from build123d import *

# Parameters (mm, degrees)
BOSS_EXTRUDE2_DEPTH = 10
SKETCH2_R           = 4
CUT_EXTRUDE1_DEPTH  = 10


with BuildPart() as part:
    # Sketch1 → Boss-Extrude2 (new body)
    with BuildSketch(Plane.XY):
        Polygon((0, 25.51264103), (0, 30), (1.000891574, 30), (10.376925968, 23.306957325), (12.202099292, 27.406363729), (13.116459243, 26.99926445), (18.959587166, 17.071288962), (22.294344764, 20.073918191), (22.96407195, 19.330110797), (24.263963499, 7.88383965), (28.531695489, 9.270509831), (28.840987995, 8.318605378), (25.372880113, -2.666797161), (29.835656861, -3.135853898), (29.731035203, -4.131262483), (22.094595249, -12.756320515), (25.980762114, -15), (25.480316326, -15.86679753), (14.995954144, -20.640160164), (17.633557569, -24.270509831), (16.823819276, -24.858819138), (5.304376334, -24.955128612), (6.237350725, -29.344428022), (5.258331033, -29.552525082), (-5.304376334, -24.955128612), (-6.237350725, -29.344428022), (-7.216370416, -29.136330963), (-14.995954144, -20.640160164), (-17.633557569, -24.270509831), (-18.443295862, -23.682200525), (-22.094595249, -12.756320515), (-25.980762114, -15), (-26.481207901, -14.13320247), (-25.372880113, -2.666797161), (-29.835656861, -3.135853898), (-29.940278519, -2.140445313), (-24.263963499, 7.88383965), (-28.531695489, 9.270509831), (-28.222402983, 10.222414285), (-18.959587165, 17.071288962), (-22.294344764, 20.073918191), (-21.624617578, 20.817725585), (-10.376925968, 23.306957325), (-12.202099292, 27.406363729), (-11.287739341, 27.813463008), align=None)
    extrude(amount=BOSS_EXTRUDE2_DEPTH)

    # Sketch2 → Cut-Extrude1 (cut)
    with BuildSketch(Plane(origin=(0, 0, 0), x_dir=(-1, 0, 0), z_dir=(0, 0, -1))):
        Circle(SKETCH2_R)
    extrude(amount=-CUT_EXTRUDE1_DEPTH, mode=Mode.SUBTRACT)


solid = part.part
The listing builds one solid part. Answer for the finished solid, in the listing's coordinates (mm). A direction names the side the tool comes from. Give positions to 0.01 mm unless a question says otherwise; leave off trailing zeros. Order: outer loops, then holes, each group sorted by start corner. A loop starts at its lowest first (then second) coordinate and runs counter-clockwise, first axis right, second up. Notation, with made-up numbers: (-35, 54) - (-16, 54) arc R24 cw to (-16, 72) - close; hole circle Ø8 at (68.25, 87). An arc over 180 degrees is marked (long way). Answer as CSV lines item,"result".
Q1. Determine the mould class of faces 1 (the face through (11.277, 25.328, 4.93)), 2 (the face through (0.051, -27.286, 4.93)), 3 (the face through (-11.277, 25.328, 4.93)), 4 (the face through (0, 28, 5)) for opening direction Y: pulls with the +Y half, pulls with the -Y half, needs draft (parallel to the pull), parting line crosses it, or undercut.
Answer key:
face 1,"pulls with the +Y half"
face 2,"pulls with the -Y half"
face 3,"undercut"
face 4,"needs draft"
Q2. A cutting plane is placed at A-A, the plane x = 16. Determine the outline of the cut face in (y, z), and give its area (3 significant figures).
Answer key:
outline,"(-24.87, 0) - (-22.02, 0) - (-22.02, 10) - (-24.87, 10) - close; (-20.18, 0) - (22.1, 0) - (22.1, 10) - (-20.18, 10) - close"
area,"451 mm^2"
Q3. A cutting plane is placed at B-B, the plane y = 0. Determine the outline of the cut face in (x, z).
Answer key:
outline,"(-28.73, 0) - (-4, 0) - (-4, 10) - (-28.73, 10) - close; (4, 0) - (26.21, 0) - (26.21, 10) - (4, 10) - close"
Q4. A cutting plane is placed at D-D, the plane y = -6.5. Determine the outline of the cut face in (x, z).
Answer key:
outline,"(-25.74, 0) - (27.63, 0) - (27.63, 10) - (-25.74, 10) - close"
Q5. Straight lines are drawn through the part: L1, parallel to Y at x = 25, z = 7.75; L2, parallel to X at y = 17.5, z = 5.5; L3, parallel to Y at x = 17, z = 7. For each, find the intervals that lie inside material, in ascending order.
Answer key:
L1,"y = -16.09 to -14.43, -9.47 to 8.12"
L2,"x = -19.44 to 18.71, 19.44 to 23.17"
L3,"y = -24.73 to -23.4, -19.73 to 20.4"
Q6. Which of the six approach directions +Z, -Z, +X, -X, +Y, -Y give full straight-line access (tool end or side, diameter ignored) to faces 5 (the face through (-27.6, -2.9, 4.9)), 6 (the face through (16, 22.1, 4.9)), 7 (the face through (16.296, -22.43, 4.93))?
Answer key:
face 5,"+Z, -Z"
face 6,"+Z, -Z, +Y"
face 7,"+Z, -Z, +X"
Q7. Each of these flat-tipped pins is pushed along its axis until it touches: pin 1 Ø6 at (x, z) = (-18.5, 8.5) entering from +Y; pin 2 Ø2 at (x, y) = (20.5, 22) entering from -Z; pin 3 Ø1 at (x, z) = (13.5, 6) entering from -Y; pin 4 Ø2 at (y, z) = (10, 5) entering from -X. Where does it stop, or does it pass through?
Answer key:
pin 1,"stops at y = 22.17"
pin 2,"passes through"
pin 3,"stops at y = -24.89"
pin 4,"stops at x = -28.53"
Q8. A cutting plane is placed at C-C, the plane x = 9. Determine the outline of the cut face in (y, z), and give its area (3 significant figures).
Answer key:
outline,"(-24.92, 0) - (24.29, 0) - (24.29, 10) - (-24.92, 10) - close"
area,"492 mm^2"
